Part print with two shaded views. Sizes in mm from the minimum x, y, z corner. A direction names the side the tool comes from. Round coordinates to 2 decimals unless told otherwise and drop trailing zeros. Write each loop counter-clockwise with the first axis right and the second up, starting at its lowest first coordinate (ties: lowest second). Pieces come first, ordered by that corner, then holes. Notation, with made-up numbers: (-10, -38.5) - (31, -38.5) arc R17 cw to (31, -18.5) - close; hole circle Ø7 at (57, -11). An arc over 180 degrees is marked (long way). Answer as a JSON object with one key per item and string values. Group by question number.
Item 1: Which spindle directions (+Z, -Z, +X, -X, +Y, -Y) get a long thin tool onto all of the face, cutting with end or side? Do the marked faces 1, 2 and 3. Say none if no direction does.
Item 2: Slice it at A-A, the plane y = 29. List the corners of the cut face in (x, z).
Item 3: Probe line 1 (X direction, y = 21.5, z = 33.5); line 2 (X direction, y = 17, z = 38.5); line 3 (X direction, y = 28, z = 11). List the from-to ranges inside material, lowest first. Write a range as from..to.
Item 4: Slice it at D-D, the plane z = 31.5. List the corners of the cut face in (x, y), then the cut area to 3 significant figures.
Item 5: Flat gauge pins, fed straight in: pin 1 (18 mm diameter, centred on x = 47, z = 27, fed in from +Y); pin 2 (8 mm diameter, centred on y = 5, z = 38, fed in from +X); pin 3 (12 mm diameter, centred on x = 91, y = 35, fed in from -Z); pin 4 (16.5 mm diameter, centred on x = 7, z = 28, fed in from +Y). Where does each tip first touch, or does it go through?
Item 6: Two-plate mould, pull along Z, no slides. Class the marked faces 4, 5 and 6: +Z half, -Z half, draft (parallel to the pull), parting line (faces both ways), or undercut.
Item 7: Slice it at B-B, the plane y = 22.5. List the corners of the cut face in (x, z), then the cut area to 3 significant figures.
Item 8: Slice it at C-C, the plane x = 107. List the corners of the cut face in (y, z).
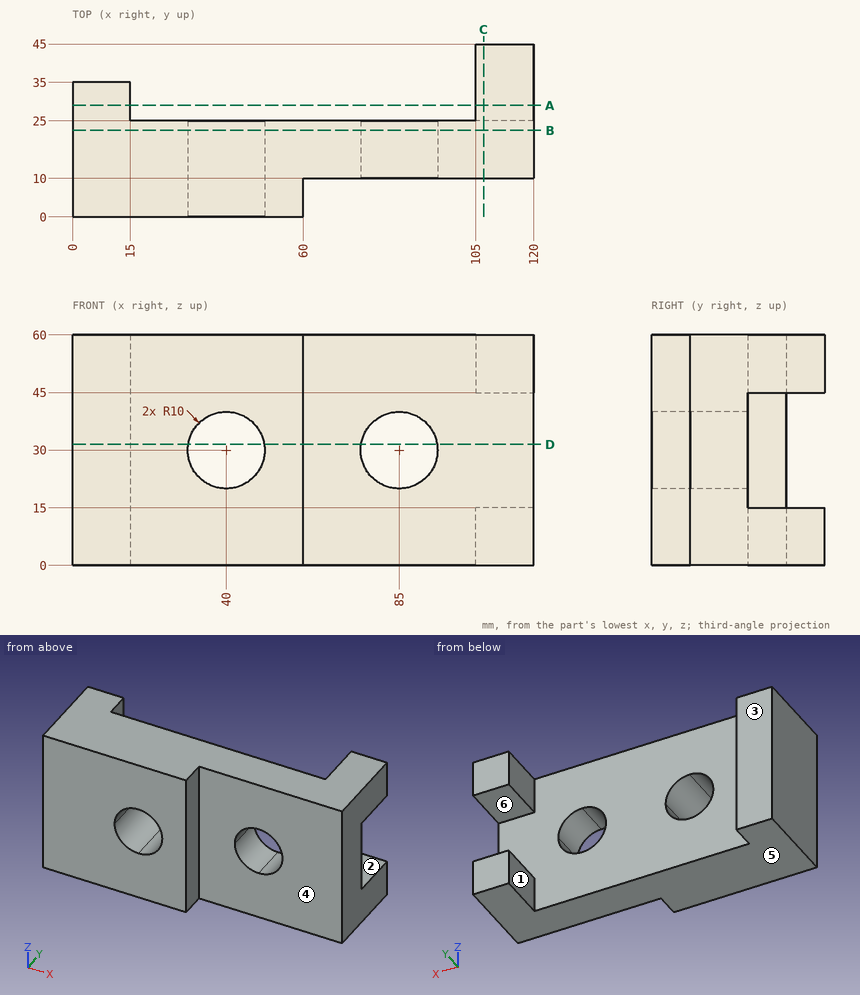
Geometry says:
{
 "1": {"face 1": "+Z, -Z, +Y", "face 2": "+X, +Y", "face 3": "+Z, -Z, -X, +Y"},
 "2": {"outline": "(0, 0) - (15, 0) - (15, 60) - (0, 60) - close; (105, 0) - (120, 0) - (120, 15) - (105, 15) - close; (105, 45) - (120, 45) - (120, 60) - (105, 60) - close"},
 "3": {"line 1": "x = 0..30.63, 49.37..75.63, 94.37..120", "line 2": "x = 0..34.73, 45.27..79.73, 90.27..120", "line 3": "x = 0..15, 105..120"},
 "4": {"outline": "(0, 0) - (30.11, 0) - (30.11, 25) - (15, 25) - (15, 35) - (0, 35) - close; (49.89, 0) - (60, 0) - (60, 10) - (75.11, 10) - (75.11, 25) - (49.89, 25) - close; (94.89, 10) - (120, 10) - (120, 25) - (94.89, 25) - close", "area": "1,760 mm^2"},
 "5": {"pin 1": "stops at y = 25", "pin 2": "stops at x = 60", "pin 3": "passes through", "pin 4": "stops at y = 35"},
 "6": {"face 4": "draft", "face 5": "-Z half", "face 6": "undercut"},
 "7": {"outline": "(0, 0) - (120, 0) - (120, 60) - (0, 60) - close; hole circle Ø20 at (40, 30); hole circle Ø20 at (85, 30)", "area": "6,570 mm^2"},
 "8": {"outline": "(10, 0) - (45, 0) - (45, 15) - (25, 15) - (25, 45) - (45, 45) - (45, 60) - (10, 60) - close"}
}
